Check sheet for the modelled part. Datum: model origin and axes. Units: mm. Round coordinates to 2 decimals unless told otherwise and drop trailing zeros. Order: outer loops, then holes, each group sorted by start corner. A loop starts at its lowest first (then second) coordinate and runs counter-clockwise, first axis right, second up.
Q1. Depth check by flat-ended pin: P1, Ø2, axis at x = 71, y = -12, coming from the -Z side. Enter the tip coordinate at first touch or a pass-through.
Q2. Cross-section at A-A on x = 21.5. Record the cut outline in (y, z).
Q3. Scan lines: probe 1 along Y at (x, z) = (107.5, 2.55); probe 2 along X at (y, z) = (-6, 1.1); probe 3 along X at (y, z) = (-4.5, 1.25). Record each from-to range of solid material in increasing order.
Q4. Cross-section at B-B on z = 0.7. Record the cut outline in (x, y), then the cut area to 3 significant figures.
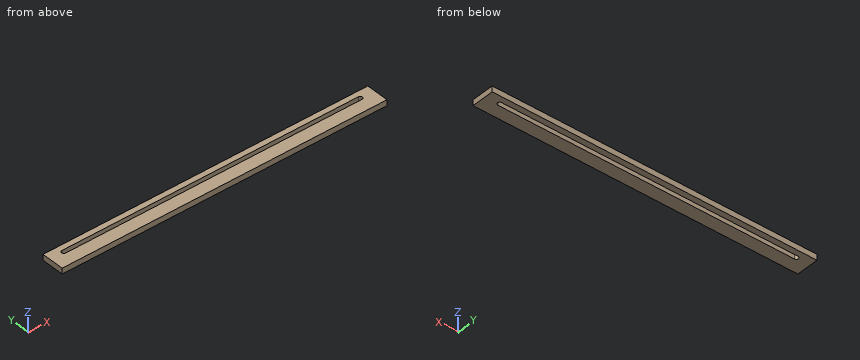
from build123d import *

# Parameters (mm, degrees)
SKETCH_1_W      = 230
SKETCH_1_H      = 16
EXTRUDE_1_DEPTH = 4


with BuildPart() as part:
    # 草图1 → 凸台-拉伸1 (new body)
    with BuildSketch(Plane.XY):
        with Locations((115, -8)):
            Rectangle(SKETCH_1_W, SKETCH_1_H)
        with BuildLine():
            Line((10, -4), (220, -4))
            ThreePointArc((220, -4), (221.5, -5.5), (220, -7))
            Line((220, -7), (10, -7))
            ThreePointArc((10, -7), (8.5, -5.5), (10, -4))
        make_face(mode=Mode.SUBTRACT)
    extrude(amount=EXTRUDE_1_DEPTH)


solid = part.part
Results found:
1. P1: stops at z = 0
2. outline: (-16, 0) - (-7, 0) - (-7, 4) - (-16, 4) - close; (-4, 0) - (0, 0) - (0, 4) - (-4, 4) - close
3. probe 1: y = -16 to -7, -4 to 0
3. probe 2: x = 0 to 8.59, 221.41 to 230
3. probe 3: x = 0 to 8.88, 221.12 to 230
4. outline: (0, -16) - (230, -16) - (230, 0) - (0, 0) - close; hole (10, -7) - (220, -7) arc R1.5 ccw to (220, -4) - (10, -4) arc R1.5 ccw to start
4. area: 3,040 mm2
